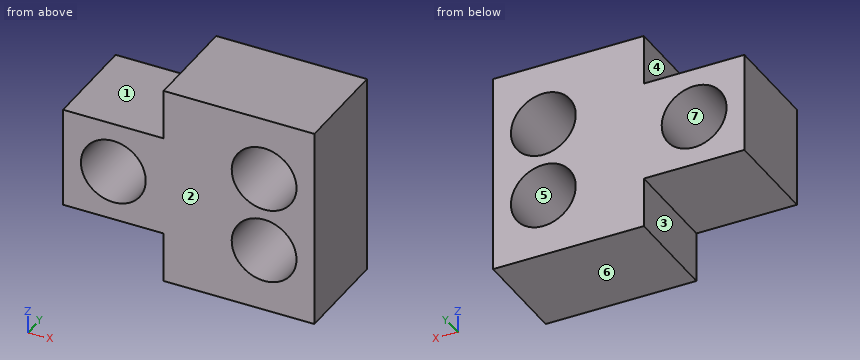
```python
from build123d import *

# Parameters (mm, degrees)
SKETCH1_R           = 6.45
SKETCH1_W           = 20
SKETCH1_H           = 20
BOSS_EXTRUDE1_DEPTH = 20


with BuildPart() as part:
    # Sketch1 → Boss-Extrude1 (new body)
    # profile 1 of 2: a face of its own
    with BuildSketch(Plane(origin=(0, 0, 0), x_dir=(1, 0, 0), z_dir=(0, 1, 0))):
        Polygon((-13.056470244, 18.913583857), (-13.056470244, 8.913583857), (-13.056470244, -11.086416143), (-13.056470244, -21.086416143), (16.943529756, -21.086416143), (16.943529756, 18.913583857), align=None)
        with Locations(Location((6.943529756, -8.586416143, 0), (0, 0, 270))):
            Circle(SKETCH1_R, mode=Mode.SUBTRACT)
        with Locations(Location((6.943529756, 6.413583857, 0), (0, 0, 270))):
            Circle(SKETCH1_R, mode=Mode.SUBTRACT)
    # profile 2 of 2: a face of its own
    with BuildSketch(Plane(origin=(0, 0, 0), x_dir=(1, 0, 0), z_dir=(0, 1, 0))):
        with Locations((-23.056470244, -1.086416143)):
            Rectangle(SKETCH1_W, SKETCH1_H)
        with Locations(Location((-23.056470244, -1.086416143, 0), (0, 0, 270))):
            Circle(SKETCH1_R, mode=Mode.SUBTRACT)
    extrude(amount=BOSS_EXTRUDE1_DEPTH)


solid = part.part
```
The listing builds one solid part. Answer for the finished solid, in the listing's coordinates (mm). Face numbers are marked on the shaded views. A direction names the side the tool comes from. Round coordinates to 2 decimals unless told otherwise and drop trailing zeros. Loops run counter-clockwise (first coordinate to the right, second up) from the corner with the lowest first, then second, coordinate; pieces in that order, holes last.
Q1. Find the intervals of material crossed by line 1 (Z direction, x = 11.5, y = 19.25); line 2 (X direction, y = 4.5, z = -2); line 3 (Z direction, x = 6, y = 17), in increasing order.
Q2. Section D-D, the plane z = 1.5 is taken. Determine the outline of the cut face in (x, y).
Q3. For a pull along Z with two mould halves and no side action, classify the marked faces 4, 5, 6 and 7 as released by +Z, released by -Z, zero draft, split by the parting line, or undercut.
Q4. Section C-C, the plane y = 16.5 is taken. Determine the outline of the cut face in (x, z).
Q5. Section B-B, the plane x = -19 is taken. Determine the outline of the cut face in (y, z), then the cut area to 3 significant figures.
Q6. Section A-A, the plane z = 5.5 is taken. Determine the outline of the cut face in (x, y), then the cut area to 3 significant figures.
Q7. Given pin 1 Ø3 at (x, y) = (-26.5, 3) entering from +Z; pin 2 Ø8 at (x, y) = (-27.5, 7) entering from -Z; pin 3 Ø3 at (y, z) = (10, -14.5) entering from -X, each flat-ended and moving along its own axis, determine where each tip first touches the part or whether it passes through.
Q8. Which of the six approach directions +Z, -Z, +X, -X, +Y, -Y give full straight-line access (tool end or side, diameter ignored) to the marked faces 1, 2 and 3?
Completed:
1. line 1: z = -18.91 to -10.98, -1.85 to 4.02, 13.15 to 21.09
1. line 2: x = -33.06 to -28.72, -17.39 to 2.24, 11.65 to 16.94
1. line 3: z = -18.91 to -12.79, -0.03 to 2.21, 14.97 to 21.09
2. outline: (-33.06, 0) - (-29.49, 0) - (-29.49, 20) - (-33.06, 20) - close; (-16.62, 0) - (16.94, 0) - (16.94, 20) - (-16.62, 20) - close
3. face 4: zero draft
3. face 5: undercut
3. face 6: released by -Z
3. face 7: undercut
4. outline: (-33.06, -8.91) - (-13.06, -8.91) - (-13.06, -18.91) - (16.94, -18.91) - (16.94, 21.09) - (-13.06, 21.09) - (-13.06, 11.09) - (-33.06, 11.09) - close; hole circle Ø12.9 at (-23.06, 1.09); hole circle Ø12.9 at (6.94, -6.41); hole circle Ø12.9 at (6.94, 8.59)
5. outline: (0, -8.91) - (20, -8.91) - (20, -3.93) - (0, -3.93) - close; (0, 6.1) - (20, 6.1) - (20, 11.09) - (0, 11.09) - close
5. area: 199 mm2
6. outline: (-33.06, 0) - (-27.76, 0) - (-27.76, 20) - (-33.06, 20) - close; (-18.35, 0) - (1.28, 0) - (1.28, 20) - (-18.35, 20) - close; (12.61, 0) - (16.94, 0) - (16.94, 20) - (12.61, 20) - close
6. area: 585 mm2
7. pin 1: stops at z = 11.09
7. pin 2: stops at z = -8.91
7. pin 3: stops at x = -13.06
8. face 1: +Z, -X, +Y, -Y
8. face 2: +Z, -Z, +X, -X, -Y
8. face 3: -Z, -X, +Y, -Y
